Geometry check sheet. Reference: drawing and pictorial views, mm from the part's lowest x, y, z. A direction names the side the tool comes from. Give positions to 0.01 mm unless a question says otherwise; leave off trailing zeros. Order: outer loops, then holes, each group sorted by start corner. A loop starts at its lowest first (then second) coordinate and runs counter-clockwise, first axis right, second up. Notation, with made-up numbers: (-11.75, 6.5) - (28.25, 6.5) arc R23 cw to (28.25, 22.5) - close; hole circle Ø11 at (76, -35.5). An arc over 180 degrees is marked (long way). Answer in a Markdown table with one row per item.
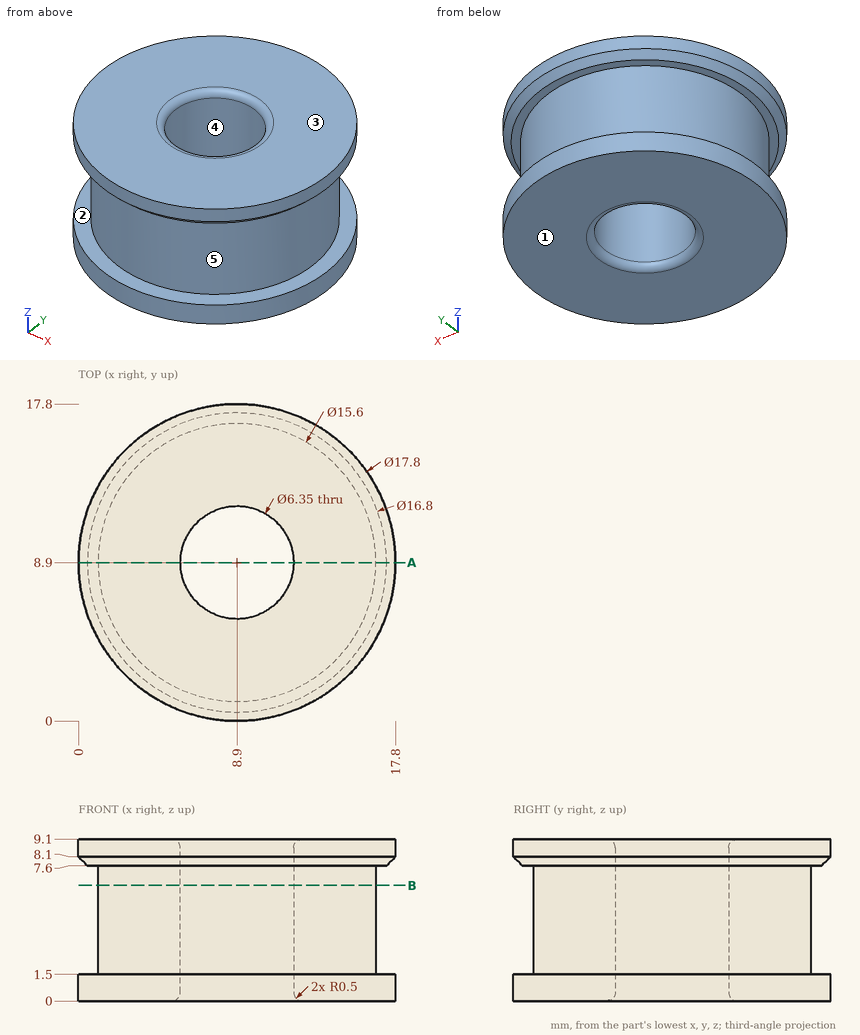
(1) Gauge pin test, flat ends, axial feed: P1, Ø2, axis at x = 13.5, z = 5, coming from the +Y side; P2, Ø4, axis at x = 8.9, y = 8.9, coming from the +Z side (3 decimals); P3, Ø1.5, axis at x = 11.5, z = 6, coming from the -Y side; P4, Ø1, axis at x = 11, z = 4, coming from the +Y side. Record the tip position at first contact, or that the pin passes through.
Geometry says:
| item | result |
|---|---|
| P1 | y = 15.82 |
| P2 | through |
| P3 | y = 1.32 |
| P4 | y = 16.53 |
(2) Thickness scan on L1, parallel to Y at x = 8.9, z = 3.5 (3 decimals); L2, parallel to X at y = 8.75, z = 7; L3, parallel to Z at x = 11.5, y = 1. Record the ranges inside material, lowest first.
Geometry says:
| item | result |
|---|---|
| L1 | 1.1 to 5.725, 12.075 to 16.7 |
| L2 | 1.1 to 5.73, 12.07 to 16.7 |
| L3 | 0 to 1.5, 7.6 to 9.1 |
(3) Cross-section at B-B, the plane z = 6.5. Record the cut outline in (x, y) (3 decimals), then the cut area to 3 significant figures.
Geometry says:
| item | result |
|---|---|
| outline | circle Ø15.6 at (8.9, 8.9); hole circle Ø6.35 at (8.9, 8.9) |
| area | 159 mm² |
(4) Cross-section at A-A, the plane y = 8.9. Record the cut outline in (x, z) (3 decimals), then the cut area to 3 significant figures.
Geometry says:
| item | result |
|---|---|
| outline | (0, 0) - (5.225, 0) arc R0.5 ccw to (5.725, 0.5) - (5.725, 8.6) arc R0.5 ccw to (5.225, 9.1) - (0, 9.1) - (0, 8.1) - (0.5, 7.6) - (1.1, 7.6) - (1.1, 1.5) - (0, 1.5) - close; (12.075, 0.5) arc R0.5 ccw to (12.575, 0) - (17.8, 0) - (17.8, 1.5) - (16.7, 1.5) - (16.7, 7.6) - (17.3, 7.6) - (17.8, 8.1) - (17.8, 9.1) - (12.575, 9.1) arc R0.5 ccw to (12.075, 8.6) - close |
| area | 90.3 mm² |
(5) Mould release check, pull along X, two halves, no side actions. Record for the marked faces 3, 4 and 5: pulls with the +X half, pulls with the -X half, needs draft (parallel to the pull), parting line crosses it, or undercut.
Geometry says:
| item | result |
|---|---|
| face 3 | needs draft |
| face 4 | undercut |
| face 5 | parting line crosses it |
(6) Access from +Z, -Z, +X, -X, +Y, -Y to the whole of each face (thin tool, end or side, straight path). Record for the marked faces 1 and 2.
Geometry says:
| item | result |
|---|---|
| face 1 | -Z, +X, -X, +Y, -Y |
| face 2 | none |
